```python
from build123d import *

# Parameters (mm, degrees)
SKETCH_1_R          = 10
EXTRUDE_1_DEPTH     = 5.5
SKETCH_2_W          = 3.6
SKETCH_2_H          = 6
EXTRUDE_2_DEPTH     = 9.7
CUT_EXTRUDE_START   = -3.6
CUT_EXTRUDE_1_DEPTH = 3.6
CHAMFER_1_SIZE      = 1
SKETCH_4_R          = 1.5
EXTRUDE_3_DEPTH     = 2


# Read off the part's stored shape, not the designer's step: 切除-拉伸1
with BuildPart() as part:
    # 草图1 → 凸台-拉伸1 (new body)
    with BuildSketch(Plane.XY):
        Circle(SKETCH_1_R)
    extrude(amount=EXTRUDE_1_DEPTH)

    # 草图2 → 凸台-拉伸2 (add)
    with BuildSketch(Plane.XY.offset(5.5)):
        Rectangle(SKETCH_2_W, SKETCH_2_H)
    extrude(amount=EXTRUDE_2_DEPTH)

    # 切除-拉伸1 outline → 切除-拉伸1 (cut)
    with BuildSketch(Plane.ZY.offset(1.8).offset(CUT_EXTRUDE_START)):
        with BuildLine():
            Line((15.2, 3), (13.113552873, 3))
            ThreePointArc((13.113552873, 3), (14.627105745, 1.827105745), (15.2, 0))
            Line((15.2, 0), (15.2, 3))
        make_face()
        with BuildLine():
            Line((15.2, -3), (15.2, 0))
            ThreePointArc((15.2, 0), (14.627105745, -1.827105745), (13.113552873, -3))
            Line((13.113552873, -3), (15.2, -3))
        make_face()
    extrude(amount=CUT_EXTRUDE_1_DEPTH, mode=Mode.SUBTRACT)

    # 倒角1
    chamfer_1_edges = [part.edges().sort_by_distance(p)[0] for p in [
        (-10, 0, 0),
    ]]
    chamfer(chamfer_1_edges, length=CHAMFER_1_SIZE)

    # 草图4 → 凸台-拉伸3 (add)
    with BuildSketch(Plane.ZY.offset(1.8)):
        with Locations(Location((12, 0, 0), (0, 0, 180))):
            Circle(SKETCH_4_R)
    extrude_3 = extrude(amount=EXTRUDE_3_DEPTH)

    # 镜向1: 凸台-拉伸3 across plane
    add(extrude_3.mirror(Plane(origin=(0, 0, 0), x_dir=(0, 0, 1), z_dir=(1, 0, 0))))


solid = part.part
```
Build history of the part. All positions in model axes, mm. A direction names the side the tool comes from. Coordinates: 2 decimals unless noted, no trailing zeros. Order: outer loops, then holes, each group sorted by start corner. A loop starts at its lowest first (then second) coordinate and runs counter-clockwise, first axis right, second up. Notation, with made-up numbers: M 6,5 L 40,5 A21 cw 40,32 Z; hole C 37.5,-24.75 d5. An arc over 180 degrees is marked long. One line per question, with ' | ' between items. Start each with the question number.
1. Wall check: line 1 along Z through (x, y) = (0.5, 6.75); line 2 along Y through (x, z) = (-1, 10.5); line 3 along X through (y, z) = (-2.5, 10.75). Give the ranges that are in metal, low to high. Write a range as [from, to].
2. Cut at B-B (x = 0). Write the cut outline in (y, z).
3. Tool access for faces 1 (the face through (3.8, 0, 12)), 2 (the face through (-2.79, -0.07, 13.5)), 3 (the face through (-3.8, 0, 12)), 4 (the face through (0, -3, 9)): list every direction of +Z, -Z, +X, -X, +Y, -Y with a clear straight run to the whole face (end or side of a thin tool).
4. Cut at D-D (z = 14). Write the cut outline in (x, y), plus the area to 3 significant figures.
5. Cut at A-A (z = 12). Write the cut outline in (x, y).
6. Mould opens along Z. For faces 5 (the face through (2.79, -0.07, 13.5)), 6 (the face through (0, 0, 0)), 7 (the face through (1.8, 0, 10)), 8 (the face through (0, 3, 9)) say: +Z half, -Z half, draft (parallel to the pull), parting line (faces both ways), or undercut.
7. Flat gauge pins, fed straight in: P1, Ø3, axis at y = -0.5, z = 11, coming from the +X side; P2, Ø4, axis at y = 5.5, z = 2, coming from the -X side; P3, Ø1.8, axis at x = -0.5, z = 8, coming from the -Y side; P4, Ø1.5, axis at y = 5, z = 8.5, coming from the -X side. Where does each tip first touch, or does it go through?
8. Cut at C-C (z = 4.25). Write the cut outline in (x, y), plus the area to 3 significant figures.
The answers:
1) line 1: z = [0, 5.5] | line 2: y = [-3, 3] | line 3: x = [-1.8, 1.8]
2) outline: M -10,1 L -9,0 L 9,0 L 10,1 L 10,5.5 L 3,5.5 L 3,13.11 A3.2 ccw -3,13.11 L -3,5.5 L -10,5.5 Z
3) face 1: +Z, +X, +Y, -Y | face 2: -X | face 3: +Z, -X, +Y, -Y | face 4: +Z, +X, -X, -Y
4) outline: M -1.8,-2.5 L 1.8,-2.5 L 1.8,2.5 L -1.8,2.5 Z | area: 18.0 mm2
5) outline: M -3.8,-1.5 L -1.8,-1.5 L -1.8,-3 L 1.8,-3 L 1.8,-1.5 L 3.8,-1.5 L 3.8,1.5 L 1.8,1.5 L 1.8,3 L -1.8,3 L -1.8,1.5 L -3.8,1.5 Z
6) face 5: undercut | face 6: -Z half | face 7: undercut | face 8: draft
7) P1: stops at x = 3.8 | P2: stops at x = -9.37 | P3: stops at y = -3 | P4: passes through
8) outline: C 0,0 d20 | area: 314 mm2
